from build123d import *

# Parameters (mm, degrees)
CROQUIS1_R              = 35
CROQUIS1_R_2            = 29
SALIENTE_EXTRUIR1_DEPTH = 8
REDONDEO1_R             = 10
CROQUIS2_R              = 2.5
CORTAR_EXTRUIR1_DEPTH   = 10


with BuildPart() as part:
    # Croquis1 → Saliente-Extruir1 (new body)
    # profile 1 of 5: a face of its own
    with BuildSketch(Plane(origin=(0, 0, 0), x_dir=(1, 0, 0), z_dir=(0, 1, 0))):
        Circle(CROQUIS1_R)
        with Locations(Location((0, 0, 0), (0, 0, 270))):
            Circle(CROQUIS1_R_2, mode=Mode.SUBTRACT)
    # profile 2 of 5: a face of its own
    with BuildSketch(Plane(origin=(0, 0, 0), x_dir=(1, 0, 0), z_dir=(0, 1, 0))):
        with BuildLine():
            ThreePointArc((-1.9e-08, -35), (-24.748737387, -24.748737296), (-35, 1.1e-07))
            Line((-35, 1.1e-07), (-35, -35))
            Line((-35, -35), (-1.9e-08, -35))
        make_face()
    # profile 3 of 5: a face of its own
    with BuildSketch(Plane(origin=(0, 0, 0), x_dir=(1, 0, 0), z_dir=(0, 1, 0))):
        with BuildLine():
            Line((35, -35), (35, 0))
            ThreePointArc((35, 0), (24.748737335, -24.748737348), (-1.9e-08, -35))
            Line((-1.9e-08, -35), (35, -35))
        make_face()
    # profile 4 of 5: a face of its own
    with BuildSketch(Plane(origin=(0, 0, 0), x_dir=(1, 0, 0), z_dir=(0, 1, 0))):
        with BuildLine():
            Line((35, 35), (1.1e-08, 35))
            ThreePointArc((1.1e-08, 35), (24.748737345, 24.748737338), (35, 0))
            Line((35, 0), (35, 35))
        make_face()
    # profile 5 of 5: a face of its own
    with BuildSketch(Plane(origin=(0, 0, 0), x_dir=(1, 0, 0), z_dir=(0, 1, 0))):
        with BuildLine():
            Line((1.1e-08, 35), (-35, 35))
            Line((-35, 35), (-35, 1.1e-07))
            ThreePointArc((-35, 1.1e-07), (-24.748737299, 24.748737384), (1.1e-08, 35))
        make_face()
    extrude(amount=SALIENTE_EXTRUIR1_DEPTH)

    # Redondeo1
    redondeo1_edges = [part.edges().sort_by_distance(p)[0] for p in [
        (-35, 4, -35),
        (35, 4, -35),
        (35, 4, 35),
        (-35, 4, 35),
    ]]
    fillet(redondeo1_edges, radius=REDONDEO1_R)

    # Croquis2 → Cortar-Extruir1 (cut)
    with BuildSketch(Plane(origin=(0, 8, 0), x_dir=(1, 0, 0), z_dir=(0, 1, 0))):
        with Locations(Location((-27, 27, 0), (0, 0, 270))):
            Circle(CROQUIS2_R)
        with Locations(Location((27, 27, 0), (0, 0, 270))):
            Circle(CROQUIS2_R)
        with Locations(Location((27, -27, 0), (0, 0, 270))):
            Circle(CROQUIS2_R)
        with Locations(Location((-27, -27, 0), (0, 0, 270))):
            Circle(CROQUIS2_R)
    extrude(amount=-CORTAR_EXTRUIR1_DEPTH, mode=Mode.SUBTRACT)


solid = part.part
The listing builds one solid part. Answer for the finished solid, in the listing's coordinates (mm). Coordinates: 2 decimals unless noted, no trailing zeros. Loops run counter-clockwise (first coordinate to the right, second up) from the corner with the lowest first, then second, coordinate; pieces in that order, holes last. Notation, with made-up numbers: (45, 85.25) -> (60, 85.25) arc R21 cw to (60, 100.25) -> close; hole circle Ø10 at (-16, 8.5). An arc over 180 degrees is marked (long way). Answer in a Markdown table with one row per item. Add a question column.
1. Determine the mould class of faces 1 (the cylindrical face through (31.99, 4.06, 32.15)), 2 (the cylindrical face through (-25.31, 4.06, -28.84)), 3 (the cylindrical face through (-31.99, 4.06, -32.15)) for opening direction X: +X half, -X half, draft (parallel to the pull), parting line (faces both ways), or undercut.
2. Consider line 1 (X direction, y = 5.75, z = 0); line 2 (X direction, y = 4.75, z = -25.5); line 3 (X direction, y = 3.25, z = -25). Determine where each line is inside the solid, lowest interval first. Write a range as [from, to].
3. The part is cut by section A-A, the plane y = 4.5. Write down the section's boundary in (x, z), then the cut area to 3 significant figures.
4. The part is cut by section D-D, the plane x = 28. Write down the section's boundary in (y, z).
5. The part is cut by section B-B, the plane z = 0. Write down the section's boundary in (x, y).
6. The part is cut by section C-C, the plane x = 17. Write down the section's boundary in (y, z).
Answer below:
| question | item | result |
|---|---|---|
| 1 | face 1 | +X half |
| 1 | face 2 | undercut |
| 1 | face 3 | -X half |
| 2 | line 1 | [-35, -29], [29, 35] |
| 2 | line 2 | [-34.99, -29], [-25, -13.81], [13.81, 25], [29, 34.99] |
| 2 | line 3 | [-35, -28.5], [-25.5, -14.7], [14.7, 25.5], [28.5, 35] |
| 3 | outline | (-35, -25) arc R10 ccw to (-25, -35) -> (25, -35) arc R10 ccw to (35, -25) -> (35, 25) arc R10 ccw to (25, 35) -> (-25, 35) arc R10 ccw to (-35, 25) -> close; hole circle Ø5 at (-27, -27); hole circle Ø5 at (-27, 27); hole circle Ø58 at (0, 0); hole circle Ø5 at (27, -27); hole circle Ø5 at (27, 27) |
| 3 | area | 2,090 mm2 |
| 4 | outline | (0, -34.54) -> (8, -34.54) -> (8, -29.29) -> (0, -29.29) -> close; (0, -24.71) -> (8, -24.71) -> (8, -7.55) -> (0, -7.55) -> close; (0, 7.55) -> (8, 7.55) -> (8, 24.71) -> (0, 24.71) -> close; (0, 29.29) -> (8, 29.29) -> (8, 34.54) -> (0, 34.54) -> close |
| 5 | outline | (-35, 0) -> (-29, 0) -> (-29, 8) -> (-35, 8) -> close; (29, 0) -> (35, 0) -> (35, 8) -> (29, 8) -> close |
| 6 | outline | (0, -35) -> (8, -35) -> (8, -23.49) -> (0, -23.49) -> close; (0, 23.49) -> (8, 23.49) -> (8, 35) -> (0, 35) -> close |
